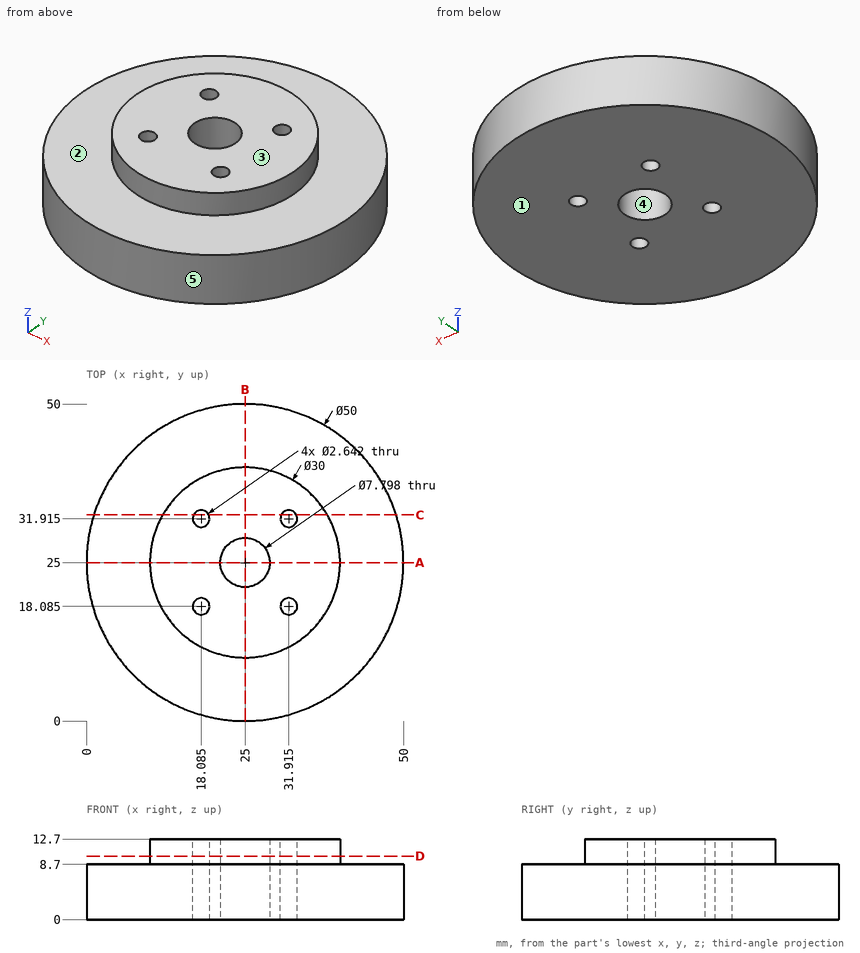
Check sheet for the drawn part. Datum: minimum x, y, z corner. Units: mm. A direction names the side the tool comes from. Give positions to 0.01 mm unless a question says otherwise; leave off trailing zeros. Order: outer loops, then holes, each group sorted by start corner. A loop starts at its lowest first (then second) coordinate and runs counter-clockwise, first axis right, second up. Notation, with made-up numbers: (49, 70) -> (64, 70) arc R19 ccw to (64, 84) -> close; hole circle Ø2 at (-16, 43.5). An arc over 180 degrees is marked (long way). Answer as CSV lines item,"result".
Q1. Sectioned sample at D-D on z = 10. Record the cut outline in (x, y) (1 decimal), plus the area to 3 significant figures.
Solutions:
outline,"circle Ø30 at (25, 25); hole circle Ø2.6 at (18.1, 18.1); hole circle Ø2.6 at (18.1, 31.9); hole circle Ø7.8 at (25, 25); hole circle Ø2.6 at (31.9, 18.1); hole circle Ø2.6 at (31.9, 31.9)"
area,"637 mm²"
Q2. Scan lines: probe 1 along Y at (x, z) = (25, 12); probe 2 along Y at (x, z) = (17.5, 3.5); probe 3 along Z at (x, y) = (27.5, 47). Record each from-to range of solid material in increasing order.
Solutions:
probe 1,"y = 10 to 21.1, 28.9 to 40"
probe 2,"y = 1.15 to 16.9, 19.27 to 30.73, 33.1 to 48.85"
probe 3,"z = 0 to 8.7"
Q3. Access from +Z, -Z, +X, -X, +Y, -Y to the whole of each face (thin tool, end or side, straight path). Record for the marked faces 1 and 2.
Solutions:
face 1,"-Z, +X, -X, +Y, -Y"
face 2,"+Z"
Q4. Sectioned sample at A-A on y = 25. Record the cut outline in (x, z), plus the area to 3 significant figures.
Solutions:
outline,"(0, 0) -> (21.1, 0) -> (21.1, 12.7) -> (10, 12.7) -> (10, 8.7) -> (0, 8.7) -> close; (28.9, 0) -> (50, 0) -> (50, 8.7) -> (40, 8.7) -> (40, 12.7) -> (28.9, 12.7) -> close"
area,"456 mm²"
Q5. Depth check by flat-ended pin: pin 1 (5 mm diameter, centred on y = 31, z = 11, fed in from -X); pin 2 (2 mm diameter, centred on x = 19, z = 9, fed in from +Y); pin 3 (6 mm diameter, centred on y = 11.5, z = 2.5, fed in from +X); pin 4 (2.5 mm diameter, centred on x = 31.91, y = 18.09, fed in from -Z). Enter the tip coordinate at first touch or a pass-through.
Solutions:
pin 1,"stops at x = 0.51"
pin 2,"stops at y = 49.49"
pin 3,"stops at x = 47.69"
pin 4,"passes through"
Q6. Sectioned sample at C-C on y = 32.5. Record the cut outline in (x, z).
Solutions:
outline,"(1.15, 0) -> (16.9, 0) -> (16.9, 12.7) -> (12.01, 12.7) -> (12.01, 8.7) -> (1.15, 8.7) -> close; (19.27, 0) -> (30.73, 0) -> (30.73, 12.7) -> (19.27, 12.7) -> close; (33.1, 0) -> (48.85, 0) -> (48.85, 8.7) -> (37.99, 8.7) -> (37.99, 12.7) -> (33.1, 12.7) -> close"
Q7. Release check for a two-part mould opening along X. For the marked faces 3, 4 and 5 record: +X half, -X half, draft (parallel to the pull), parting line (faces both ways), or undercut.
Solutions:
face 3,"draft"
face 4,"undercut"
face 5,"parting line"
